```python
from build123d import *

# Parameters (mm, degrees)
SKETCH1_R           = 25
SKETCH1_R_2         = 1.85
SKETCH1_R_3         = 5
BOSS_EXTRUDE1_DEPTH = 6
SKETCH2_R           = 12.5
SKETCH2_R_2         = 5
BOSS_EXTRUDE2_DEPTH = 11
SKETCH3_R           = 10
SKETCH3_R_2         = 5
BOSS_EXTRUDE3_DEPTH = 20
FILLET1_R           = 5
SKETCH4_W           = 6.35
SKETCH4_H           = 6.35
CUT_EXTRUDE1_DEPTH  = 4


with BuildPart() as part:
    # Sketch1 → Boss-Extrude1 (new body)
    with BuildSketch(Plane.XY):
        Circle(SKETCH1_R)
        with Locations((-13.029498672, -13.274798425)):
            Circle(SKETCH1_R_2, mode=Mode.SUBTRACT)
        with Locations((13.029498672, -13.274798425)):
            Circle(SKETCH1_R_2, mode=Mode.SUBTRACT)
        with Locations((13.029498672, 13.274798425)):
            Circle(SKETCH1_R_2, mode=Mode.SUBTRACT)
        with Locations((-13.029498672, 13.274798425)):
            Circle(SKETCH1_R_2, mode=Mode.SUBTRACT)
        Circle(SKETCH1_R_3, mode=Mode.SUBTRACT)
    extrude(amount=BOSS_EXTRUDE1_DEPTH)

    # Sketch2 → Boss-Extrude2 (add)
    with BuildSketch(Plane.XY.offset(6)):
        Circle(SKETCH2_R)
        Circle(SKETCH2_R_2, mode=Mode.SUBTRACT)
    extrude(amount=BOSS_EXTRUDE2_DEPTH)

    # Sketch3 → Boss-Extrude3 (add)
    with BuildSketch(Plane.XY.offset(17)):
        Circle(SKETCH3_R)
        Circle(SKETCH3_R_2, mode=Mode.SUBTRACT)
    extrude(amount=BOSS_EXTRUDE3_DEPTH)

    # Fillet1
    fillet1_edges = [part.edges().sort_by_distance(p)[0] for p in [
        (-10, 0, 37),
    ]]
    fillet(fillet1_edges, radius=FILLET1_R - 0.0001)  # a hair under: the kernel refuses the full size

    # Sketch4 → Cut-Extrude1 (cut)
    with BuildSketch(Plane.XY.offset(6)):
        with Locations((13.029498672, -13.274798425)):
            Rectangle(SKETCH4_W, SKETCH4_H)
        with Locations((13.029498672, 13.274798425)):
            Rectangle(SKETCH4_W, SKETCH4_H)
        with Locations((-13.029498672, 13.274798425)):
            Rectangle(SKETCH4_W, SKETCH4_H)
        with Locations((-13.029498672, -13.274798425)):
            Rectangle(SKETCH4_W, SKETCH4_H)
    extrude(amount=-CUT_EXTRUDE1_DEPTH, mode=Mode.SUBTRACT)


solid = part.part
```
Work out the finished part from the listing and answer in its coordinate system (mm). A direction names the side the tool comes from. Round coordinates to 2 decimals unless told otherwise and drop trailing zeros. Order: outer loops, then holes, each group sorted by start corner. A loop starts at its lowest first (then second) coordinate and runs counter-clockwise, first axis right, second up.
Q1. A cutting plane is placed at D-D, the plane y = -14. Determine the outline of the cut face in (x, z).
Solution:
outline: (-20.71, 0) - (-14.73, 0) - (-14.73, 2) - (-16.2, 2) - (-16.2, 6) - (-20.71, 6) - close; (-11.33, 0) - (11.33, 0) - (11.33, 2) - (9.85, 2) - (9.85, 6) - (-9.85, 6) - (-9.85, 2) - (-11.33, 2) - close; (14.73, 0) - (20.71, 0) - (20.71, 6) - (16.2, 6) - (16.2, 2) - (14.73, 2) - close
Q2. Given pin 1 Ø4.5 at (x, z) = (-13.5, 3.5) entering from -Y; pin 2 Ø6 at (x, y) = (1, 17.5) entering from +Z; pin 3 Ø4.5 at (y, z) = (-13.5, 3.5) entering from +X; pin 4 Ø7.5 at (x, y) = (0, 1) entering from +Z, each flat-ended and moving along its own axis, determine where each tip first touches the part or whether it passes through.
Solution:
pin 1: stops at y = -22.33
pin 2: stops at z = 6
pin 3: stops at x = 22.33
pin 4: passes through
Q3. The mould has two halves that part along X. Classify faces 3 (the flat face through (-13, -16.45, 4)), 4 (the flat face through (-0.3, -5.2, 0)): pulls with the +X half, pulls with the -X half, needs draft (parallel to the pull), parting line crosses it, or undercut.
Solution:
face 3: undercut
face 4: needs draft
Q4. A cutting plane is placed at C-C, the plane z = 18. Determine the outline of the cut face in (x, y), then the cut area to 3 significant figures.
Solution:
outline: circle Ø20 at (0, 0); hole circle Ø10 at (0, 0)
area: 236 mm2
Q5. Find the intervals of material crossed by line 1 along X through (y, z) = (13, 5.5); line 2 along Z through (x, y) = (-12.5, -4.5); line 3 along Y through (x, z) = (0, 22.5), in increasing order.
Solution:
line 1: x = -21.35 to -16.2, -9.85 to 9.85, 16.2 to 21.35
line 2: z = 0 to 6
line 3: y = -10 to -5, 5 to 10
Q6. A tool of negligible diameter and unlimited length cuts with its end or side. For faces 1 (the cylindrical face through (14.74, -13.98, 0.99)), 2 (the flat face through (9.854, 13, 4)), from which of +Z, -Z, +X, -X, +Y, -Y can it reach the whole face along a straight path? Write none if from no direction.
Solution:
face 1: +Z, -Z
face 2: +Z
